Work out the finished part from the listing and answer in its coordinate system (mm). Face numbers are marked on the shaded views. Round coordinates to 2 decimals unless told otherwise and drop trailing zeros. Write each loop counter-clockwise with the first axis right and the second up, starting at its lowest first coordinate (ties: lowest second). Pieces come first, ordered by that corner, then holes. Notation, with made-up numbers: (71.25, 29.5) -> (130.25, 29.5) arc R28 ccw to (130.25, 60.5) -> close; hole circle Ø1 at (63, 32.5). An arc over 180 degrees is marked (long way). Answer as a JSON object with one key per item and string values. Group by question number.
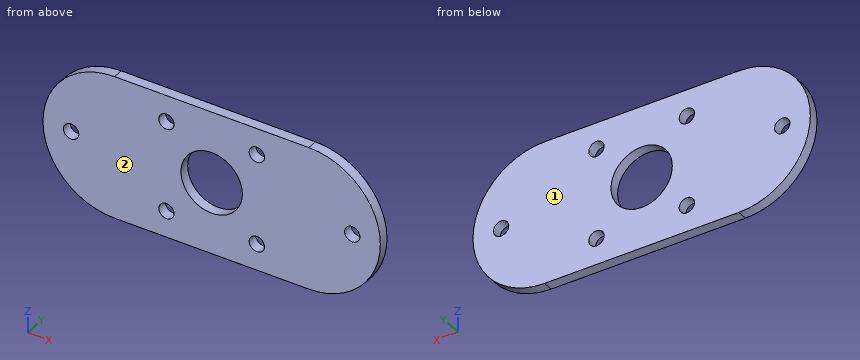
Autodesk Inventor part; units mm, degrees
ref_plane "YZ Plane" through (0, 0, 0) normal (1, 0, 0) x (0, 1, 0)
ref_plane "XZ Plane" through (0, 0, 0) normal (0, 1, 0) x (-1, 0, 0)
ref_plane "XY Plane" through (0, 0, 0) normal (0, 0, 1) x (1, 0, 0)
sketch "Sketch2" plane through (0, 0, 0) normal (0, 1, 0) x (-1, 0, 0)
  line L0 (0, 0) -> (28, 0)
  line L1 (28, 0) -> (28, -28)
  line L2 (28, -28) -> (0, -28)
  line L3 (0, -28) -> (0, 0)
  line L4 (28, 0) -> (0, -28) construction
  line L5 (28, -28) -> (0, 0) construction
  circle A0 centre (22.8388, -5.1612) radius 1.5
  circle A1 centre (22.8388, -22.8388) radius 1.5
  circle A2 centre (5.1612, -5.1612) radius 1.5
  circle A3 centre (5.1612, -22.8388) radius 1.5
  circle A4 centre (14, -14) radius 6
  line L6 (28, -28) -> (33, -28)
  line L7 (33, -28) -> (33, 0)
  line L8 (33, 0) -> (28, 0)
  line L9 (28, 0) -> (28, -28)
  line L10 (0, -28) -> (-5, -28)
  line L11 (-5, -28) -> (-5, 0)
  line L12 (-5, 0) -> (0, 0)
  line L13 (0, 0) -> (0, -28)
  arc A5 (33, -28) -> (33, 0) centre (33, -14) ccw
  arc A6 (-5, 0) -> (-5, -28) centre (-5, -14) ccw
  circle A7 centre (41.5, -14) radius 1.5
  circle A8 centre (-13.5, -14) radius 1.5
  dimension "d37" = 3
  dimension "d38" = 3
  dimension "d39" = 3
  dimension "d40" = 3
  dimension "d41" = 12.5
  dimension "d42" = 12.5
  dimension "d43" = 12.5
  dimension "d44" = 12.5
  dimension "d60" = 28
  dimension "d61" = 12
  dimension "d66" = 5
  dimension "d67" = 5
  dimension "d68" = 3
  dimension "d69" = 3
  dimension "d70" = 8.5
  dimension "d71" = 8.5
extrude "Extrusion2" add sketch "Sketch2" along normal blind 2
sketch "Sketch3" plane through (0, 2, 0) normal (0, 1, 0) x (1, 0, 0)
  line L0 (5, 28) -> (-33, 28)
  arc A0 (-33, 28) -> (-33, 0) centre (-33, 14) ccw
  line L1 (-33, 0) -> (5, 0)
  arc A1 (5, 0) -> (5, 28) centre (5, 14) ccw
  circle A2 centre (-22.8388, 22.8388) radius 1.5
  circle A3 centre (-5.1612, 5.1612) radius 1.5
  circle A4 centre (-14, 14) radius 6
  circle A5 centre (-5.1612, 22.8388) radius 1.5
  circle A6 centre (-22.8388, 5.1612) radius 1.5
  circle A7 centre (-41.5, 14) radius 1.5
  circle A8 centre (13.5, 14) radius 1.5
  point P0 (0, 0)
properties part number "Motor_mount_plate_large"
1) A cutting plane is placed at A-A on x = -14. Determine the outline of the cut face in (y, z).
2) For a pull along Y with two mould halves and no side action, classify the marked faces 1 and 2 as released by +Y, released by -Y, zero draft, split by the parting line, or undercut.
3) Straight lines are drawn through the part: L1, parallel to X at y = 0.15, z = -6.5; L2, parallel to X at y = 1.55, z = -4.5; L3, parallel to Z at x = -14, y = 1.55. For each, find the intervals that lie inside material, in ascending order.
4) A cutting plane is placed at C-C on y = 0.35. Determine the outline of the cut face in (x, z).
5) A cutting plane is placed at B-B on z = -14. Determine the outline of the cut face in (x, y), plus the area to 3 significant figures.
6) A cutting plane is placed at D-D on z = -17.5. Determine the outline of the cut face in (x, y).
7) Each of these flat-tipped pins is pushed along its axis until it touches: P1, Ø4, axis at x = -41.5, z = -14, coming from the +Y side; P2, Ø1.8, axis at x = -22.84, z = -5.16, coming from the +Y side. Where does it stop, or does it pass through?
Established:
{
 "1": {"outline": "(0, -28) -> (2, -28) -> (2, -20) -> (0, -20) -> close; (0, -8) -> (2, -8) -> (2, 0) -> (0, 0) -> close"},
 "2": {"face 1": "released by +Y", "face 2": "released by -Y"},
 "3": {"L1": "x = -44.82 to -23.52, -22.16 to -5.84, -4.48 to 16.82", "L2": "x = -43.28 to -24.19, -21.49 to -6.51, -3.81 to 15.28", "L3": "z = -28 to -20, -8 to 0"},
 "4": {"outline": "(-33, -28) -> (5, -28) arc R14 ccw to (5, 0) -> (-33, 0) arc R14 ccw to start; hole circle Ø3 at (-41.5, -14); hole circle Ø3 at (-22.84, -22.84); hole circle Ø3 at (-22.84, -5.16); hole circle Ø12 at (-14, -14); hole circle Ø3 at (-5.16, -22.84); hole circle Ø3 at (-5.16, -5.16); hole circle Ø3 at (13.5, -14)"},
 "5": {"outline": "(-47, 0) -> (-43, 0) -> (-43, 2) -> (-47, 2) -> close; (-40, 0) -> (-20, 0) -> (-20, 2) -> (-40, 2) -> close; (-8, 0) -> (12, 0) -> (12, 2) -> (-8, 2) -> close; (15, 0) -> (19, 0) -> (19, 2) -> (15, 2) -> close", "area": "96.0 mm²"},
 "6": {"outline": "(-46.56, 0) -> (-18.87, 0) -> (-18.87, 2) -> (-46.56, 2) -> close; (-9.13, 0) -> (18.56, 0) -> (18.56, 2) -> (-9.13, 2) -> close"},
 "7": {"P1": "stops at y = 2", "P2": "passes through"}
}
